The model under review builds one solid part; all positions refer to its coordinate system, in mm. Face numbers are marked on the shaded views. A direction names the side the tool comes from. Coordinates: 2 decimals unless noted, no trailing zeros. Order: outer loops, then holes, each group sorted by start corner. A loop starts at its lowest first (then second) coordinate and runs counter-clockwise, first axis right, second up. Notation, with made-up numbers: M -22,6.5 L 21,6.5 A13 cw 21,30.5 Z; hole C 1.5,-40 d5. An arc over 180 degrees is marked long. Write each question's results on one line, items separated by ' | '.
from build123d import *

# Parameters (mm, degrees)
SKETCH2_R                   = 100
BOSS_EXTRUDE1_DEPTH         = 3
SKETCH3_R                   = 7.5
BOSS_EXTRUDE2_DEPTH         = 4.75
CIRPATTERN1_COUNT           = 5
FILLET3_R                   = 8
SKETCH5_R                   = 1
CUT_EXTRUDE1_DEPTH          = 3
BOSS_EXTRUDE3_DEPTH         = 3
TAP_DRILL_FOR_M4X0_7_TAP1_D = 3.3
TAP_DRILL_FOR_M4X0_7_TAP2_D = 3.3
SKETCH10_R                  = 1
CUT_EXTRUDE2_DEPTH          = 142.633550056


with BuildPart() as part:
    # Sketch2 → Boss-Extrude1 (new body)
    with BuildSketch(Plane(origin=(0, 0, 0), x_dir=(1, 0, 0), z_dir=(0, 1, 0))):
        with Locations(Location((0, 0, 0), (0, 0, 270))):
            Circle(SKETCH2_R)
    extrude(amount=BOSS_EXTRUDE1_DEPTH)

    # Sketch3 → Boss-Extrude2 (add)
    with BuildSketch(Plane.XZ):
        with Locations(Location((0, 75, 0), (0, 0, 90))):
            Circle(SKETCH3_R)
    boss_extrude2 = extrude(amount=BOSS_EXTRUDE2_DEPTH)

    # CirPattern1: Boss-Extrude2 ×5 about axis
    cirpattern1_axis = Axis((0, 0, 0), (0, 1, 0))
    for i in range(1, CIRPATTERN1_COUNT):
        add(boss_extrude2.rotate(cirpattern1_axis, i * 360 / CIRPATTERN1_COUNT))

    # Fillet3
    # the kernel refuses this fillet: 8 mm, written as the material it takes off along each edge
    with BuildSketch(Plane(origin=(-71.329238722, -4.75, 23.176274578), x_dir=(-0.9510565162951535, 0, 0.30901699437494723), z_dir=(0.30901699437494723, 0, 0.9510565162951535))) as fillet3_piece_1:
        with BuildLine():
            CenterArc((0.189904241, -8), FILLET3_R, 23.969482318, 66.030517682)
            Line((0.189904241, 0), (0.189904241, 0.16))
            Line((0.189904241, 0.16), (7.5, 0.16))
            Line((7.5, 0.16), (7.66, 0))
            ThreePointArc((7.66, 0), (7.66, -2.375), (7.646201915, -4.685))
            Line((7.646201915, -4.685), (7.5, -4.75))
        make_face()
    revolve(axis=Axis((-71.329238722, -4.75, 23.176274578), (0, -1, 0)), mode=Mode.SUBTRACT)
    with BuildSketch(Plane(origin=(-44.083893922, -4.75, -60.676274578), x_dir=(-0.5877852522924734, 0, -0.8090169943749472), z_dir=(-0.8090169943749472, 0, 0.5877852522924734))) as fillet3_piece_2:
        with BuildLine():
            CenterArc((0.189904241, -8), FILLET3_R, 23.969482318, 66.030517682)
            Line((0.189904241, 0), (0.189904241, 0.16))
            Line((0.189904241, 0.16), (7.5, 0.16))
            Line((7.5, 0.16), (7.66, 0))
            ThreePointArc((7.66, 0), (7.66, -2.375), (7.646201915, -4.685))
            Line((7.646201915, -4.685), (7.5, -4.75))
        make_face()
    revolve(axis=Axis((-44.083893922, -4.75, -60.676274578), (0, -1, 0)), mode=Mode.SUBTRACT)
    with BuildSketch(Plane(origin=(44.083893922, -4.75, -60.676274578), x_dir=(0.5877852522924734, 0, -0.8090169943749472), z_dir=(-0.8090169943749472, 0, -0.5877852522924734))) as fillet3_piece_3:
        with BuildLine():
            CenterArc((0.189904241, -8), FILLET3_R, 23.969482318, 66.030517682)
            Line((0.189904241, 0), (0.189904241, 0.16))
            Line((0.189904241, 0.16), (7.5, 0.16))
            Line((7.5, 0.16), (7.66, 0))
            ThreePointArc((7.66, 0), (7.66, -2.375), (7.646201915, -4.685))
            Line((7.646201915, -4.685), (7.5, -4.75))
        make_face()
    revolve(axis=Axis((44.083893922, -4.75, -60.676274578), (0, -1, 0)), mode=Mode.SUBTRACT)
    with BuildSketch(Plane(origin=(71.329238722, -4.75, 23.176274578), x_dir=(0.9510565162951535, 0, 0.30901699437494723), z_dir=(0.30901699437494723, 0, -0.9510565162951535))) as fillet3_piece_4:
        with BuildLine():
            CenterArc((0.189904241, -8), FILLET3_R, 23.969482318, 66.030517682)
            Line((0.189904241, 0), (0.189904241, 0.16))
            Line((0.189904241, 0.16), (7.5, 0.16))
            Line((7.5, 0.16), (7.66, 0))
            ThreePointArc((7.66, 0), (7.66, -2.375), (7.646201915, -4.685))
            Line((7.646201915, -4.685), (7.5, -4.75))
        make_face()
    revolve(axis=Axis((71.329238722, -4.75, 23.176274578), (0, -1, 0)), mode=Mode.SUBTRACT)
    with BuildSketch(Plane(origin=(0, -4.75, 75), x_dir=(0, 0, 1), z_dir=(1, 0, 0))) as fillet3_piece_5:
        with BuildLine():
            CenterArc((0.189904241, -8), FILLET3_R, 23.969482318, 66.030517682)
            Line((0.189904241, 0), (0.189904241, 0.16))
            Line((0.189904241, 0.16), (7.5, 0.16))
            Line((7.5, 0.16), (7.66, 0))
            ThreePointArc((7.66, 0), (7.66, -2.375), (7.646201915, -4.685))
            Line((7.646201915, -4.685), (7.5, -4.75))
        make_face()
    revolve(axis=Axis((0, -4.75, 75), (0, -1, 0)), mode=Mode.SUBTRACT)

    # Sketch5 → Cut-Extrude1 (cut)
    with BuildSketch(Plane.XZ):
        with Locations(Location((0, 8, 0), (0, 0, 270))):
            Circle(SKETCH5_R)
        with Locations(Location((5.656854249, 5.656854249, 0), (0, 0, 270))):
            Circle(SKETCH5_R)
        with Locations(Location((8, 0, 0), (0, 0, 270))):
            Circle(SKETCH5_R)
        with Locations(Location((5.656854249, -5.656854249, 0), (0, 0, 270))):
            Circle(SKETCH5_R)
        with Locations(Location((0, -8, 0), (0, 0, 270))):
            Circle(SKETCH5_R)
        with Locations(Location((-5.656854249, -5.656854249, 0), (0, 0, 270))):
            Circle(SKETCH5_R)
        with Locations(Location((-8, 0, 0), (0, 0, 270))):
            Circle(SKETCH5_R)
        with Locations(Location((-5.656854249, 5.656854249, 0), (0, 0, 270))):
            Circle(SKETCH5_R)
    extrude(amount=-CUT_EXTRUDE1_DEPTH, mode=Mode.SUBTRACT)

    # Sketch5<3> → Boss-Extrude3 (add)
    with BuildSketch(Plane.XZ):
        with BuildLine():
            Line((0.75, -9.5), (-0.75, -9.5))
            Line((-0.75, -9.5), (-0.75, -10.974402034))
            ThreePointArc((-0.75, -10.974402034), (0, -11), (0.75, -10.974402034))
            Line((0.75, -10.974402034), (0.75, -9.5))
        make_face()
        with BuildLine():
            ThreePointArc((0.75, -10.974402034), (0, -11), (-0.75, -10.974402034))
            Line((-0.75, -10.974402034), (-0.75, -12.5))
            Line((-0.75, -12.5), (0.75, -12.5))
            Line((0.75, -12.5), (0.75, -10.974402034))
        make_face()
    extrude(amount=BOSS_EXTRUDE3_DEPTH)

    # Tap Drill for M4x0.7 Tap1 (through all)
    with Locations(Plane(origin=(-45, 3, -30), x_dir=(0, 0, 1), z_dir=(0, 1, 0))):
        with Locations((0, 0), (0, 30), (60, 0), (60, 30)):
            Hole(TAP_DRILL_FOR_M4X0_7_TAP1_D / 2)

    # Tap Drill for M4x0.7 Tap2 (through all)
    with Locations(Plane(origin=(15, 3, -27.6), x_dir=(0, 0, 1), z_dir=(0, 1, 0))):
        with Locations((0, 0), (60, 0), (60, 50), (0, 50)):
            Hole(TAP_DRILL_FOR_M4X0_7_TAP2_D / 2)

    # Sketch10 → Cut-Extrude2 (cut, through all)
    with BuildSketch(Plane(origin=(0, 3, 0), x_dir=(1, 0, 0), z_dir=(0, 1, 0))):
        with Locations(Location((5, -55, 0), (0, 0, 270))):
            Circle(SKETCH10_R)
        with Locations(Location((-5, -55, 0), (0, 0, 270))):
            Circle(SKETCH10_R)
    extrude(amount=-CUT_EXTRUDE2_DEPTH, mode=Mode.SUBTRACT)


solid = part.part
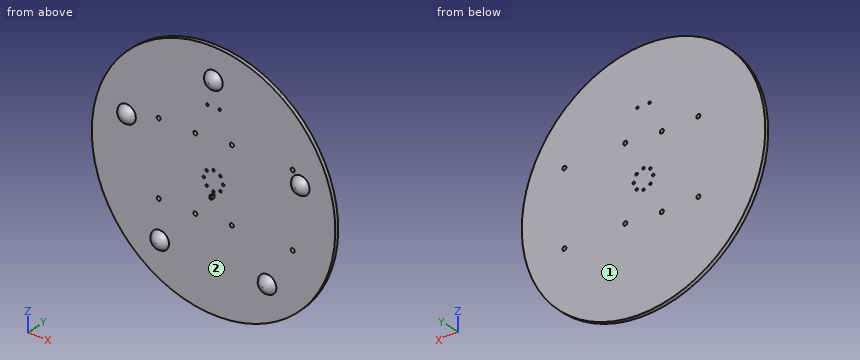
1) To check wall thickness, follow line 1 along X through (y, z) = (1.05, -30); line 2 along X through (y, z) = (2.35, 0); line 3 along Y through (x, z) = (29.5, 24). State the ranges of each line that lie inside material, in increasing order.
Solutions:
line 1: -95.39 to -46.65, -43.35 to -16.65, -13.35 to 95.39 | line 2: -100 to -9, -7 to 7, 9 to 100 | line 3: 0 to 3
2) Take a section at A-A on y = 1.5. Count the separate pieces of the cut face and the enclosed holes in it, plus the area to 3 significant figures.
Solutions:
separate pieces: 1 | enclosed holes: 18 | area: 31,300 mm2
3) Take a section at B-B on x = -87.5. State the section outline as (y, z) points, plus the area to 3 significant figures.
Solutions:
outline: M 0,-48.41 L 3,-48.41 L 3,48.41 L 0,48.41 Z | area: 290 mm2
4) For the marked faces 1 and 2, list the 3-axis set-ups (+Z, -Z, +X, -X, +Y, -Y) from which the entire face can be reached by the end or side of a thin tool; tool diameter is ignored.
Solutions:
face 1: +Z, -Z, +X, -X, +Y | face 2: -Y
5) For pin 1 (4 mm diameter, centred on x = -16, z = -80, fed in from -Y); pin 2 (2.5 mm diameter, centred on y = -1, z = -10.5, fed in from -X); pin 3 (1.5 mm diameter, centred on y = -1.5, z = -11, fed in from +X), all flat-tipped, find the tip position at first contact; note any pin that passes through.
Solutions:
pin 1: y = 0 | pin 2: x = -99.52 | pin 3: x = 0.75
6) Take a section at C-C on z = 60. State the section outline as (x, y) points.
Solutions:
outline: M -80,0 L 80,0 L 80,3 L -80,3 Z
